Can you work these out from the model? Positions are in its coordinate system, mm. A direction names the side the tool comes from. Give positions to 0.01 mm unless a question says otherwise; leave off trailing zeros. Loops run counter-clockwise (first coordinate to the right, second up) from the corner with the lowest first, then second, coordinate; pieces in that order, holes last. Notation, with made-up numbers: (52, 62) - (91, 62) arc R30 ccw to (91, 99) - close; hole circle Ø4 at (-7.5, 79.25). An arc over 180 degrees is marked (long way). Answer as a JSON object with one key per item and string values. Group by question number.
Item 1: Suppose I cut it at B-B on z = 0. Write out the boundary of the cut face in (x, y).
Item 2: Please list where these lines run through material, in increasing order: L1, parallel to Y at x = 16, z = 1.5; L2, parallel to Z at x = 1.75, y = 1.75; L3, parallel to Z at x = 20, y = 0.5.
Item 3: Suppose I cut it at C-C on y = 3.75. Write out the boundary of the cut face in (x, z), and give its area (3 significant figures).
Item 4: Will these pins go through, and if not, where does the flat tip stop? pin 1 (5 mm diameter, centred on y = 0.1, z = 18.2, fed in from +X); pin 2 (5 mm diameter, centred on y = -1.5, z = 19, fed in from +X); pin 3 (5 mm diameter, centred on y = 0, z = 0, fed in from -X); pin 4 (4.5 mm diameter, centred on x = 16, y = 0, fed in from +Z).
Item 5: Suppose I cut it at A-A on x = 16. Write out the boundary of the cut face in (y, z).
Item 6: Which directions (+Z, -Z, +X, -X, +Y, -Y) give clear straight access to the entire face, cutting with the end or side of a thin tool? Please do faces 1 (the flat face through (13.5, 0, 8.055)), 2 (the flat face through (9, 5.104, 0)), 3 (the cylindrical face through (5, -2, 0)), 4 (the flat face through (7, 0.2, -14.7)), 5 (the flat face through (2, 0, -26)).
Item 7: Thinking about a two-plate mould opening in X: for faces 6 (the flat face through (9, -4.896, 0)), 7 (the flat face through (24, 0, 0)), 8 (the cylindrical face through (14.4, -1.2, 0.2)), which applies, pulls with the +X half, pulls with the -X half, needs draft (parallel to the pull), parting line crosses it, or undercut?
Item 8: Suppose I cut it at D-D on x = 2.5. Write out the boundary of the cut face in (y, z), and give its area (3 significant figures).
from build123d import *

# Parameters (mm, degrees)
SKETCH_1_W                    = 52
SKETCH_1_H                    = 10
EXTRUDE_1_DEPTH               = 24
SKETCH_2_W                    = 23.570504403
SKETCH_2_H                    = 14.285983016
SKETCH_2_W_2                  = 23.570504402
CUT_EXTRUDE_1_DEPTH           = 17
FILLET_1_R                    = 1
CHAMFER_1_SIZE                = 2
SKETCH_3_R                    = 2
CUT_EXTRUDE_2_DEPTH           = 32.480923073
SKETCH_4_R                    = 2
CUT_EXTRUDE_3_DEPTH           = 42.973818432
SKETCH_5_R                    = 3
CUT_EXTRUDE_4_DEPTH           = 2
CUT_EXTRUDE_4_DRAFT           = -27
CUT_EXTRUDE_4_PROFILE_2_DEPTH = 2
CUT_EXTRUDE_4_PROFILE_2_DRAFT = -27
SKETCH_6_R                    = 2
CUT_EXTRUDE_2_2_DEPTH         = 10


with BuildPart() as part:
    # Эскиз1 → Вытянуть1 (new body)
    with BuildSketch(Plane(origin=(0, 0, 0), x_dir=(0, 0, -1), z_dir=(1, 0, 0))):
        with Locations((0, 0.103774831)):
            Rectangle(SKETCH_1_W, SKETCH_1_H)
    extrude(amount=EXTRUDE_1_DEPTH)

    # Эскиз2 → Вырез-Вытянуть1 (cut)
    with BuildSketch(Plane(origin=(24, 0, 0), x_dir=(0, 0, -1), z_dir=(1, 0, 0))):
        with Locations((-19.840397425, -1.378733322)):
            Rectangle(SKETCH_2_W, SKETCH_2_H)
        with Locations((19.730106978, -1.378733322)):
            Rectangle(SKETCH_2_W_2, SKETCH_2_H)
    extrude(amount=-CUT_EXTRUDE_1_DEPTH, mode=Mode.SUBTRACT)

    # Скругление1
    fillet_1_edges = [part.edges().sort_by_distance(p)[0] for p in [
        (7, 0.103774831, 8.055145223),
        (7, 0.103774831, -7.944854777),
    ]]
    fillet(fillet_1_edges, radius=FILLET_1_R)

    # Фаска1
    chamfer_1_edges = [part.edges().sort_by_distance(p)[0] for p in [
        (24, 0.103774831, 8.055145223),
        (7, 0.103774831, 26),
        (24, 0.103774831, -7.944854777),
        (7, 0.103774831, -26),
    ]]
    chamfer(chamfer_1_edges, length=CHAMFER_1_SIZE)

    # Эскиз3 → Cut-Extrude 2 (cut, through all)
    with BuildSketch(Plane(origin=(7, 0, 0), x_dir=(0, 0, -1), z_dir=(1, 0, 0))):
        with Locations((-18.202696524, 0.103774831)):
            Circle(SKETCH_3_R)
        with Locations((18.092406077, 0.103774831)):
            Circle(SKETCH_3_R)
    extrude(amount=-CUT_EXTRUDE_2_DEPTH, mode=Mode.SUBTRACT)

    # Эскиз4 → Вырез-Вытянуть3 (cut, through all)
    with BuildSketch(Plane.XY.offset(8.055145223)):
        with Locations((16, 0)):
            Circle(SKETCH_4_R)
    extrude(amount=-CUT_EXTRUDE_3_DEPTH, mode=Mode.SUBTRACT)


with BuildPart() as cut_extrude_4_tool:
    # Эскиз5 → Вырез-Вытянуть4 (with draft: the straight prism first)
    with BuildSketch(Plane(origin=(7, 0, 0), x_dir=(0, 0, -1), z_dir=(1, 0, 0))):
        with Locations((-18.202696524, 0.103774831)):
            Circle(SKETCH_5_R)
    extrude(amount=-CUT_EXTRUDE_4_DEPTH)
    # Вырез-Вытянуть4: the draft: its side faces are tilted about the plane it starts from
    cut_extrude_4_sides = [cut_extrude_4_tool.faces().sort_by_distance(p)[0] for p in [
        (6, 0.103774831, 21.202696524),
    ]]
    draft(cut_extrude_4_sides, Plane(origin=(7, 0, 0), x_dir=(0, 0, -1), z_dir=(1, 0, 0)), CUT_EXTRUDE_4_DRAFT)


with BuildPart() as part_1:
    add(part.part)

    # Вырез-Вытянуть4: cut by cut_extrude_4_tool
    add(cut_extrude_4_tool.part, mode=Mode.SUBTRACT)


with BuildPart() as cut_extrude_4_profile_2_tool:
    # Эскиз5 → Вырез-Вытянуть4 profile 2 (with draft: the straight prism first)
    with BuildSketch(Plane(origin=(7, 0, 0), x_dir=(0, 0, -1), z_dir=(1, 0, 0))):
        with Locations((18.092406077, 0.103774831)):
            Circle(SKETCH_5_R)
    extrude(amount=-CUT_EXTRUDE_4_PROFILE_2_DEPTH)
    # Вырез-Вытянуть4 profile 2: the draft: its side faces are tilted about the plane it starts from
    cut_extrude_4_profile_2_sides = [cut_extrude_4_profile_2_tool.faces().sort_by_distance(p)[0] for p in [
        (6, 0.103774831, -15.092406077),
    ]]
    draft(cut_extrude_4_profile_2_sides, Plane(origin=(7, 0, 0), x_dir=(0, 0, -1), z_dir=(1, 0, 0)), CUT_EXTRUDE_4_PROFILE_2_DRAFT)


with BuildPart() as part_2:
    add(part_1.part)

    # Вырез-Вытянуть4 profile 2: cut by cut_extrude_4_profile_2_tool
    add(cut_extrude_4_profile_2_tool.part, mode=Mode.SUBTRACT)

    # Эскиз6 → Cut-Extrude 2 2 (cut)
    with BuildSketch(Plane.ZY):
        Circle(SKETCH_6_R)
    extrude(amount=-CUT_EXTRUDE_2_2_DEPTH, mode=Mode.SUBTRACT)


solid = part_2.part
Worked out:
{
 "1": {"outline": "(0, -4.9) - (24, -4.9) - (24, 5.1) - (0, 5.1) - (0, 2) - (10, 2) - (10, -2) - (0, -2) - close; hole circle Ø4 at (16, 0)"},
 "2": {"L1": "y = -4.9 to -2, 2 to 5.1", "L2": "z = -26 to -19.23, -16.96 to -0.97, 0.97 to 17.07, 19.34 to 26", "L3": "z = -7.94 to 8.06"},
 "3": {"outline": "(0, -26) - (5, -26) - (7, -24) - (7, -8.94) arc R1 cw to (8, -7.94) - (22, -7.94) - (24, -5.94) - (24, 6.06) - (22, 8.06) - (8, 8.06) arc R1 cw to (7, 9.06) - (7, 24) - (5, 26) - (0, 26) - close", "area": "628 mm2"},
 "4": {"pin 1": "stops at x = 6.03", "pin 2": "stops at x = 7", "pin 3": "stops at x = 0", "pin 4": "stops at z = 8.06"},
 "5": {"outline": "(-4.9, -7.94) - (-2, -7.94) - (-2, 8.06) - (-4.9, 8.06) - close; (2, -7.94) - (5.1, -7.94) - (5.1, 8.06) - (2, 8.06) - close"},
 "6": {"face 1": "+Z, +X, +Y, -Y", "face 2": "+Z, -Z, +X, -X, +Y", "face 3": "-X", "face 4": "-Z, +X, +Y, -Y", "face 5": "-Z, +X, -X, +Y, -Y"},
 "7": {"face 6": "needs draft", "face 7": "pulls with the +X half", "face 8": "undercut"},
 "8": {"outline": "(-4.9, -26) - (5.1, -26) - (5.1, 26) - (-4.9, 26) - close; hole circle Ø4 at (0, 0); hole circle Ø4 at (0.1, -18.09); hole circle Ø4 at (0.1, 18.2)", "area": "482 mm2"}
}
